The listing builds one solid part. Answer for the finished solid, in the listing's coordinates (mm). A direction names the side the tool comes from. Round coordinates to 2 decimals unless told otherwise and drop trailing zeros. Loops run counter-clockwise (first coordinate to the right, second up) from the corner with the lowest first, then second, coordinate; pieces in that order, holes last. Notation, with made-up numbers: (-14, 74) - (-4, 74) arc R14 ccw to (-4, 79) - close; hole circle Ø3 at (75, 8.25). An arc over 180 degrees is marked (long way). One line per question, with ' | ' between items. Start each with the question number.
from build123d import *

# Parameters (mm, degrees)
ESQUISSE2_W             = 5.361902648
ESQUISSE2_H             = 1.25
ENL_V_MAT_EXTRU_1_DEPTH = 3
ESQUISSE4_W             = 1.25
ESQUISSE4_H             = 4.5
ENL_V_MAT_EXTRU_2_DEPTH = 2.75
CHANFREIN1_SIZE         = 0.5


with BuildPart() as part:
    # Esquisse1 → Révolution1 (revolve)
    with BuildSketch(Plane.XY):
        with BuildLine():
            Line((2.754069716, 1), (3.556624327, 1))
            Line((3.556624327, 1), (5, 3.5))
            Line((5, 3.5), (7, 3.5))
            Line((7, 3.5), (7, 1.5))
            Line((7, 1.5), (13, 1.5))
            Line((13, 1.5), (13, 0))
            Line((13, 0), (-2.93, 0))
            ThreePointArc((-2.93, 0), (-0.507678901, 2.885682265), (2.754069716, 1))
        make_face()
    revolve(axis=Axis((13, 0, 0), (-1, 0, 0)))

    # Esquisse2 → Enlèv. mat.-Extru.1 (cut)
    with BuildSketch(Plane(origin=(7, 0, 0), x_dir=(0, 0, -1), z_dir=(1, 0, 0))):
        with Locations((0, 2.875)):
            Rectangle(ESQUISSE2_W, ESQUISSE2_H)
        with Locations((0, -2.875)):
            Rectangle(ESQUISSE2_W, ESQUISSE2_H)
    extrude(amount=-ENL_V_MAT_EXTRU_1_DEPTH, mode=Mode.SUBTRACT)

    # Esquisse4 → Enlèv. mat.-Extru.2 (cut)
    with BuildSketch(Plane(origin=(7, 0, 0), x_dir=(0, 0, -1), z_dir=(1, 0, 0))):
        with Locations((2.875, 0)):
            Rectangle(ESQUISSE4_W, ESQUISSE4_H)
        with Locations((-2.875, 0)):
            Rectangle(ESQUISSE4_W, ESQUISSE4_H)
    extrude(amount=-ENL_V_MAT_EXTRU_2_DEPTH, mode=Mode.SUBTRACT)

    # Chanfrein1
    chanfrein1_edges = [part.edges().sort_by_distance(p)[0] for p in [
        (13, -1.5, 0),
    ]]
    chamfer(chanfrein1_edges, length=CHANFREIN1_SIZE)


solid = part.part
(1) Each of these flat-tipped pins is pushed along its axis until it touches: P1, Ø1.4, axis at x = 5, z = -0.5, coming from the -Y side; P2, Ø3, axis at x = 8, z = 1.5, coming from the +Y side; P3, Ø2, axis at y = -1.5, z = 1.5, coming from the -X side. Where does it stop, or does it pass through?
(2) Find section C-C on x = 10.5. Write down the section's boundary in (y, z), plus the area to 3 significant figures.
(3) Find section A-A on z = 0. Write down the section's boundary in (x, y).
(4) Determine the mould class of faces 1 (the cylindrical face through (3, 0, 1)), 2 (the cylindrical face through (9.79, -1.5, -0.07)), 3 (the flat face through (13, 0, 0)), 4 (the conical face through (3.635, -0.838, -0.768)) for opening direction X: pulls with the +X half, pulls with the -X half, needs draft (parallel to the pull), parting line crosses it, or undercut.
(5) Find section D-D on y = -2.45. Write down the section's boundary in (x, z), plus the area to 3 significant figures.
(6) A tool of negligible diameter and unlimited length cuts with its end or side. For faces 5 (the flat face through (6, 2.25, 0)), 6 (the flat face through (6, -2.25, 0)), 7 (the flat face through (6, 0, 2.25)), 8 (the flat face through (7, -2, 0)), 9 (the flat face through (6, 0, -2.25)), from which of +Z, -Z, +X, -X, +Y, -Y can it reach the whole face along a straight path? Write none if from no direction.
(7) Consider L1, parallel to Y at x = 6, z = 2.05; L2, parallel to X at y = -1.85, z = 0.45; L3, parallel to X at y = 0.65, z = 1.7. Determine where each line is inside the solid, lowest interval first.
Answer below:
1) P1: y = -2.25 | P2: y = 2.25 | P3: x = -2.71
2) outline: circle Ø3 at (0, 0) | area: 7.07 mm2
3) outline: (2.75, -1) - (3.56, -1) - (4.28, -2.25) - (7, -2.25) - (7, -1.5) - (12.5, -1.5) - (13, -1) - (13, 1) - (12.5, 1.5) - (7, 1.5) - (7, 2.25) - (4.28, 2.25) - (3.56, 1) - (2.75, 1) arc R2.93 ccw (long way) to start
4) face 1: undercut | face 2: needs draft | face 3: pulls with the +X half | face 4: undercut
5) outline: circle Ø3.21 at (0, 0) | area: 8.11 mm2
6) face 5: +Z, -Z, +X, +Y | face 6: +Z, -Z, +X, -Y | face 7: +Z, +X, +Y, -Y | face 8: +X | face 9: -Z, +X, +Y, -Y
7) L1: -2.25 to 2.25 | L2: -2.23 to 2.23, 4.08 to 7 | L3: -2.3 to 2.3, 4.03 to 7
